```python
from build123d import *

# Parameters (mm, degrees)
SKETCH_1_W          = 8
SKETCH_1_H          = 8
SKETCH_1_R          = 3.05
EXTRUDE_1_DEPTH     = 8.8
SKETCH_2_W          = 8
SKETCH_2_H          = 4.5
EXTRUDE_2_DEPTH     = 8.8
SKETCH_3_R          = 3.05
CUT_EXTRUDE_1_DEPTH = 11.792590051
SKETCH_4_W          = 8
SKETCH_4_H          = 0.8
CUT_EXTRUDE_2_DEPTH = 11.792590051
SKETCH_5_W          = 2.614851978
SKETCH_5_H          = 0.8
CUT_EXTRUDE_3_DEPTH = 6
SKETCH_8_W          = 8
SKETCH_8_H          = 8
EXTRUDE_3_DEPTH     = 8
FILLET_2_R          = 2


with BuildPart() as part:
    # 草圖1 → 填料-伸長1 (new body)
    with BuildSketch(Plane(origin=(0, 0, 0), x_dir=(1, 0, 0), z_dir=(0, 1, 0))):
        Rectangle(SKETCH_1_W, SKETCH_1_H)
        with Locations(Location((0, 0, 0), (0, 0, 270))):
            Circle(SKETCH_1_R, mode=Mode.SUBTRACT)
    extrude(amount=EXTRUDE_1_DEPTH)

    # 草圖2 → 填料-伸長2 (add)
    with BuildSketch(Plane(origin=(0, 0, -4), x_dir=(-1, 0, 0), z_dir=(0, 0, -1))):
        with Locations((0, 11.05)):
            Rectangle(SKETCH_2_W, SKETCH_2_H)
    extrude(amount=-EXTRUDE_2_DEPTH)

    # 草圖3 → 除料-伸長1 (cut, through all)
    with BuildSketch(Plane.XZ.offset(-8.8)):
        with Locations(Location((0, 0, 0), (0, 0, 270))):
            Circle(SKETCH_3_R)
    extrude(amount=-CUT_EXTRUDE_1_DEPTH, mode=Mode.SUBTRACT)

    # 草圖4 → 除料-伸長2 (cut, through all)
    with BuildSketch(Plane.XZ.offset(-8.8)):
        with Locations((0, 4.4)):
            Rectangle(SKETCH_4_W, SKETCH_4_H)
    extrude(amount=-CUT_EXTRUDE_2_DEPTH, mode=Mode.SUBTRACT)

    # 草圖5 → 除料-伸長3 (cut)
    with BuildSketch(Plane.ZY.offset(4)):
        with Locations((0, 12.4)):
            Rectangle(SKETCH_5_W, SKETCH_5_H)
    extrude(amount=-CUT_EXTRUDE_3_DEPTH, mode=Mode.SUBTRACT)

    # 草圖8 → 填料-伸長3 (add)
    with BuildSketch(Plane(origin=(0, 13.3, 0), x_dir=(1, 0, 0), z_dir=(0, 1, 0))):
        Rectangle(SKETCH_8_W, SKETCH_8_H)
    extrude(amount=EXTRUDE_3_DEPTH)

    # 圓角2
    fillet_2_edges = [part.edges().sort_by_distance(p)[0] for p in [
        (4, 10.65, 4),
        (-4, 10.65, 4),
        (-4, 10.65, -4),
        (4, 10.65, -4),
    ]]
    fillet(fillet_2_edges, radius=FILLET_2_R)


solid = part.part
```
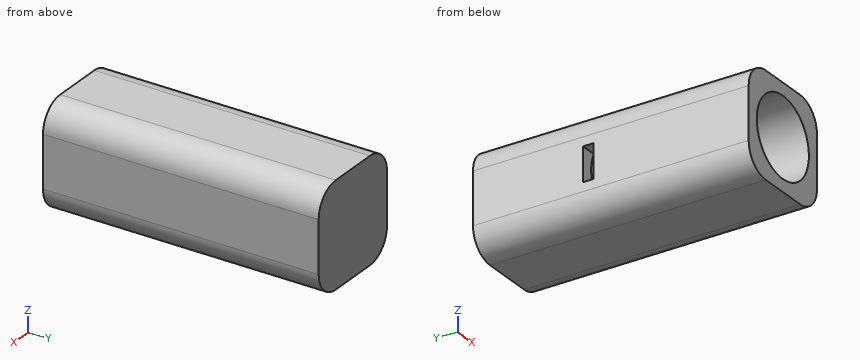
Can you work these out from the model? Positions are in its coordinate system, mm. Round coordinates to 2 decimals unless told otherwise and drop trailing zeros. Loops run counter-clockwise (first coordinate to the right, second up) from the corner with the lowest first, then second, coordinate; pieces in that order, holes last.
Item 1: Will this pin go through, and if not, where does the flat tip stop? pin 1 Ø0.9 at (x, y) = (-3.5, 12) entering from -Z.
Item 2: Suppose I cut it at B-B, the plane z = -0.75. Write out the boundary of the cut face in (x, y), then the cut area to 3 significant figures.
Item 3: Suppose I cut it at D-D, the plane y = 14. Write out the boundary of the cut face in (x, z).
Item 4: Suppose I cut it at C-C, the plane x = 0. Write out the boundary of the cut face in (y, z), then the cut area to 3 significant figures.
Item 5: Suppose I cut it at A-A, the plane y = 4. Write out the boundary of the cut face in (x, z).
Item 6: Please list where these lines run through material, in increasing order: L1, parallel to X at y = 10.95, z = 0; L2, parallel to X at y = 4.75, z = 2.5.
Reported:
1. pin 1: stops at z = -3.7
2. outline: (-4, 0) - (-2.96, 0) - (-2.96, 12) - (-4, 12) - close; (-4, 12.8) - (-2.96, 12.8) - (-2.96, 13.3) - (2.96, 13.3) - (2.96, 0) - (4, 0) - (4, 21.3) - (-4, 21.3) - close
2. area: 90.9 mm2
3. outline: (-4, -2) arc R2 ccw to (-2, -4) - (2, -4) arc R2 ccw to (4, -2) - (4, 2) arc R2 ccw to (2, 4) - (-2, 4) arc R2 ccw to (-4, 2) - close
4. outline: (0, -4) - (21.3, -4) - (21.3, 4) - (0, 4) - (0, 3.05) - (13.3, 3.05) - (13.3, -3.05) - (0, -3.05) - close
4. area: 89.3 mm2
5. outline: (-4, -2) arc R2 ccw to (-2, -4) - (2, -4) arc R2 ccw to (4, -2) - (4, 2) arc R2 ccw to (2, 4) - (-2, 4) arc R2 ccw to (-4, 2) - close; hole circle Ø6.1 at (0, 0)
6. L1: x = -4 to -3.05, 3.05 to 4
6. L2: x = -3.94 to -1.75, 1.75 to 3.94
